The model under review builds one solid part; all positions refer to its coordinate system, in mm. Face numbers are marked on the shaded views. Round coordinates to 2 decimals unless told otherwise and drop trailing zeros. Write each loop counter-clockwise with the first axis right and the second up, starting at its lowest first coordinate (ties: lowest second). Pieces come first, ordered by that corner, then holes. Notation, with made-up numbers: (38, -15.75) -> (58, -15.75) arc R30 cw to (58, 14.25) -> close; hole circle Ø7 at (57.5, 56.25). An arc over 180 degrees is marked (long way). Answer in a Markdown table with one row per item. Add a question column.
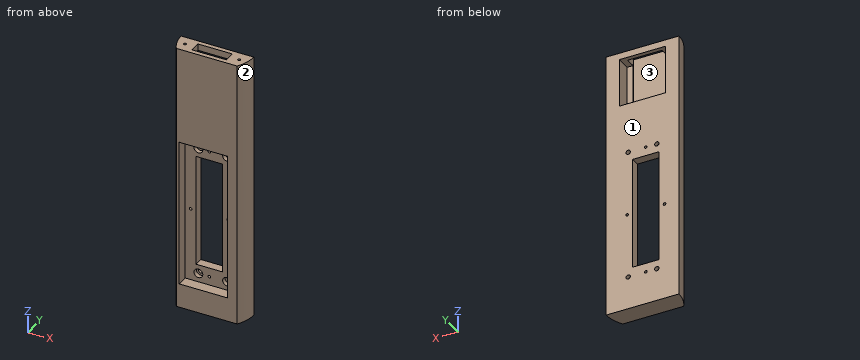
```python
from build123d import *

# Parameters (mm, degrees)
SKETCH_1_W          = 33
SKETCH_1_H          = 122
EXTRUDE_1_DEPTH     = 9
SKETCH_2_W          = 12
SKETCH_2_H          = 51
SKETCH_2_W_2        = 21
SKETCH_2_H_2        = 22
CUT_EXTRUDE_1_DEPTH = 127.70438035
SKETCH_2_2_W        = 21
SKETCH_2_2_H        = 22
EXTRUDE_2_DEPTH     = 2.5
SKETCH_3_W          = 22
SKETCH_3_H          = 67
CUT_EXTRUDE_2_DEPTH = 5
SKETCH_4_R          = 1
CUT_EXTRUDE_3_DEPTH = 127.483200466
SKETCH_4_3_R        = 2
CUT_EXTRUDE_4_DEPTH = 2
SKETCH_5_R          = 0.6
CUT_EXTRUDE_5_DEPTH = 127.483200466
SKETCH_6_OUTSIDE_W  = 60.34
SKETCH_6_OUTSIDE_H  = 36.34
SKETCH_6_OUTSIDE_R  = 16.5
CUT_EXTRUDE_6_DEPTH = 127.70438035
CUT_EXTRUDE_7_REACH = 128.704
SKETCH_7_W          = 15.6
SKETCH_7_H          = 5
SKETCH_7_3_R        = 0.6
CUT_EXTRUDE_8_DEPTH = 3


with BuildPart() as part:
    # 草图1 → 凸台-拉伸1 (new body)
    with BuildSketch(Plane(origin=(0, 0, 0), x_dir=(1, 0, 0), z_dir=(0, 1, 0))):
        with Locations((16.5, -61)):
            Rectangle(SKETCH_1_W, SKETCH_1_H)
    extrude(amount=EXTRUDE_1_DEPTH)

    # 草图2 → 切除-拉伸1 (cut, through all)
    with BuildSketch(Plane.XZ):
        with Locations((15, 44.5)):
            Rectangle(SKETCH_2_W, SKETCH_2_H)
        with Locations((16.5, 108)):
            Rectangle(SKETCH_2_W_2, SKETCH_2_H_2)
    extrude(amount=-CUT_EXTRUDE_1_DEPTH, mode=Mode.SUBTRACT)

    # 草图2<2> → 凸台-拉伸2 (add)
    with BuildSketch(Plane.XZ):
        with Locations((16.5, 108)):
            Rectangle(SKETCH_2_2_W, SKETCH_2_2_H)
    extrude(amount=-EXTRUDE_2_DEPTH)

    # 草图3 → 切除-拉伸2 (cut)
    with BuildSketch(Plane.XZ):
        with Locations((15, 44.5)):
            Rectangle(SKETCH_3_W, SKETCH_3_H)
    extrude(amount=-CUT_EXTRUDE_2_DEPTH, mode=Mode.SUBTRACT)

    # 草图4 → 切除-拉伸3 (cut, through all)
    with BuildSketch(Plane.XZ.offset(-5)):
        with Locations(Location((23, 74, 0), (0, 0, 270))):
            Circle(SKETCH_4_R)
        with Locations(Location((10, 74, 0), (0, 0, 270))):
            Circle(SKETCH_4_R)
        with Locations(Location((23, 15, 0), (0, 0, 270))):
            Circle(SKETCH_4_R)
        with Locations(Location((10, 15, 0), (0, 0, 270))):
            Circle(SKETCH_4_R)
    extrude(amount=-CUT_EXTRUDE_3_DEPTH, mode=Mode.SUBTRACT)

    # 草图4<3> → 切除-拉伸4 (cut)
    with BuildSketch(Plane.XZ.offset(-5)):
        with Locations(Location((10, 74, 0), (0, 0, 270))):
            Circle(SKETCH_4_3_R)
        with Locations(Location((23, 74, 0), (0, 0, 270))):
            Circle(SKETCH_4_3_R)
        with Locations(Location((23, 15, 0), (0, 0, 270))):
            Circle(SKETCH_4_3_R)
        with Locations(Location((10, 15, 0), (0, 0, 270))):
            Circle(SKETCH_4_3_R)
    extrude(amount=-CUT_EXTRUDE_4_DEPTH, mode=Mode.SUBTRACT)

    # 草图5 → 切除-拉伸5 (cut, through all)
    with BuildSketch(Plane.XZ.offset(-5)):
        with Locations(Location((15, 74, 0), (0, 0, 270))):
            Circle(SKETCH_5_R)
        with Locations(Location((6.5, 44.5, 0), (0, 0, 270))):
            Circle(SKETCH_5_R)
        with Locations(Location((23.5, 44.5, 0), (0, 0, 270))):
            Circle(SKETCH_5_R)
        with Locations(Location((15, 15, 0), (0, 0, 270))):
            Circle(SKETCH_5_R)
    extrude(amount=-CUT_EXTRUDE_5_DEPTH, mode=Mode.SUBTRACT)

    # 草图6 outside → 切除-拉伸6 (cut, through all)
    with BuildSketch(Plane.XY.offset(122)):
        with Locations((16.5, 4.5)):
            Rectangle(SKETCH_6_OUTSIDE_W, SKETCH_6_OUTSIDE_H)
        with Locations((16.5, 9)):
            Circle(SKETCH_6_OUTSIDE_R, mode=Mode.SUBTRACT)
    extrude(amount=-CUT_EXTRUDE_6_DEPTH, mode=Mode.SUBTRACT)

    # 切除-拉伸7: up to this face of the body (flat: up to its plane)
    cut_extrude_7_end = Plane(part.part.faces().sort_by_distance((16.5, 5.75, 97))[0])
    # 草图7 → 切除-拉伸7 (cut, up to the picked face)
    with BuildSketch(Plane.XY.offset(122), mode=Mode.PRIVATE) as cut_extrude_7_sk1:
        with Locations((16.5, 4.5)):
            Rectangle(SKETCH_7_W, SKETCH_7_H)
    cut_extrude_7_tool1 = split(extrude(cut_extrude_7_sk1.sketch, amount=-CUT_EXTRUDE_7_REACH, mode=Mode.PRIVATE), bisect_by=cut_extrude_7_end, keep=Keep.BOTH, mode=Mode.PRIVATE)
    add(cut_extrude_7_tool1.solids().sort_by(Axis((16.5, 4.5, 122), (0, 0, -1)))[0], mode=Mode.SUBTRACT)

    # 草图7<3> → 切除-拉伸8 (cut)
    with BuildSketch(Plane.XY.offset(122)):
        with Locations((4.2, 4.5)):
            Circle(SKETCH_7_3_R)
        with Locations((28.8, 4.5)):
            Circle(SKETCH_7_3_R)
    extrude(amount=-CUT_EXTRUDE_8_DEPTH, mode=Mode.SUBTRACT)


solid = part.part
```
1. Add section C-C on z = 81. Write out the cut boundary in (x, y).
2. For L1, parallel to X at y = 8.1, z = 15; L2, parallel to Z at x = 24.5, y = 2.25; L3, parallel to X at y = 8.25, z = 29, list the stretches that pass through material, from the lowest coordinate up.
3. Mouldability with a two-part tool opening along X and no side actions: class the marked faces 1, 2 and 3 as pulls with the +X half, pulls with the -X half, needs draft (parallel to the pull), parting line crosses it, or undercut.
4. Add section A-A on z = 37. Write out the cut boundary in (x, y).
5. Insertion check: pin 1 Ø1.5 at (y, z) = (3, 40.5) entering from -X; pin 2 Ø1.5 at (y, z) = (4.5, 112.5) entering from -X; pin 3 Ø1 at (y, z) = (1.5, 28.5) entering from +X. Each pin has a flat end and moves straight along its axis. Give the tip position at first contact, or say it passes through.
6. Add section B-B on x = 17. Write out the cut boundary in (y, z), plus the area to 3 significant figures.
Filled in:
| question | item | result |
|---|---|---|
| 1 | outline | (0, 9) arc R16.5 ccw to (2.67, 0) -> (30.33, 0) arc R16.5 ccw to (33, 9) -> close |
| 2 | L1 | 0.02 to 9, 11 to 14.4, 15.6 to 22, 24 to 32.98 |
| 2 | L2 | 0 to 11, 78 to 122 |
| 2 | L3 | 0.02 to 9, 21 to 32.98 |
| 3 | face 1 | needs draft |
| 3 | face 2 | pulls with the +X half |
| 3 | face 3 | undercut |
| 4 | outline | (0, 9) arc R16.5 ccw to (2.67, 0) -> (4, 0) -> (4, 5) -> (9, 5) -> (9, 9) -> close; (21, 5) -> (26, 5) -> (26, 0) -> (30.33, 0) arc R16.5 ccw to (33, 9) -> (21, 9) -> close |
| 5 | pin 1 | x = 0.86 |
| 5 | pin 2 | x = 0.43 |
| 5 | pin 3 | x = 31.44 |
| 6 | outline | (0, 0) -> (9, 0) -> (9, 19) -> (5, 19) -> (5, 11) -> (0, 11) -> close; (0, 78) -> (5, 78) -> (5, 70) -> (9, 70) -> (9, 97) -> (2, 97) -> (2, 122) -> (0, 122) -> close; (7, 119) -> (9, 119) -> (9, 122) -> (7, 122) -> close |
| 6 | area | 390 mm² |
